Check sheet for the modelled part. Datum: model origin and axes. Units: mm. Face numbers are marked on the shaded views. Round coordinates to 2 decimals unless told otherwise and drop trailing zeros. Loops run counter-clockwise (first coordinate to the right, second up) from the corner with the lowest first, then second, coordinate; pieces in that order, holes last. Notation, with made-up numbers: (-9.5, 28) -> (34.5, 28) arc R16 ccw to (34.5, 36) -> close; hole circle Ø8 at (34.25, -21.75). An arc over 180 degrees is marked (long way). One line per item, written item: value. Start each with the question number.
1. Cross-section at C-C on x = 254.5. Record the cut outline in (y, z), then the cut area to 3 significant figures.
2. Cross-section at B-B on z = 916.5. Record the cut outline in (x, y) (1 decimal).
3. Cross-section at D-D on x = 0. Record the cut outline in (y, z).
4. Material ranges on L1, parallel to Z at x = -1.5, y = 0.05; L2, parallel to Z at x = 63, y = -1.2; L3, parallel to Z at x = 177, y = 0.05, recorded low to high.
5. Go/stop test with flat-tipped pins: pin 1 (1.5 mm diameter, centred on x = 325, y = 0, fed in from +Z); pin 2 (1.6 mm diameter, centred on y = 0.5, z = 890, fed in from +X). Record where each tip stops, or that it passes through.
6. Cross-section at A-A on y = -0.25. Record the cut outline in (x, z) (3 decimals), then the cut area to 3 significant figures.
7. Release check for a two-part mould opening along Y. For the marked faces 1 and 2 record: +Y half, -Y half, draft (parallel to the pull), parting line (faces both ways), or undercut.
from build123d import *

# Parameters (mm, degrees)
BOSS_EXTRUDE1_DEPTH = 1.5875


with BuildPart() as part:
    # Sketch1 → Boss-Extrude1 (new, symmetric)
    with BuildSketch(Plane(origin=(0, 0, 0), x_dir=(1, 0, 0), z_dir=(0, 1, 0))):
        with BuildLine():
            Line((60.325, -1117.6), (525.1196, -749.3))
            Line((525.1196, -749.3), (525.1196, -647.7))
            Line((525.1196, -647.7), (-73.025, -647.7))
            Line((-73.025, -647.7), (-73.025, -1117.6))
            Line((-73.025, -1117.6), (-13.081, -1117.6))
            ThreePointArc((-13.081, -1117.6), (0, -1104.519), (13.081, -1117.6))
            Line((13.081, -1117.6), (60.325, -1117.6))
        make_face()
        Polygon((60.325, -1028.7), (60.325, -704.85), (404.076843973, -704.85), (404.076843973, -756.313435837), align=None, mode=Mode.SUBTRACT)
    extrude(amount=BOSS_EXTRUDE1_DEPTH, both=True)


solid = part.part
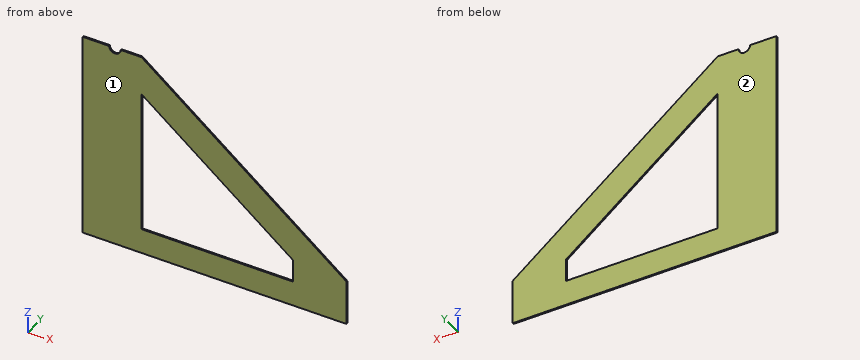
Taken from the geometry:
1. outline: (-1.59, 647.7) -> (1.59, 647.7) -> (1.59, 704.85) -> (-1.59, 704.85) -> close; (-1.59, 874.84) -> (1.59, 874.84) -> (1.59, 963.74) -> (-1.59, 963.74) -> close
1. area: 464 mm2
2. outline: (-73, -1.6) -> (60.3, -1.6) -> (60.3, 1.6) -> (-73, 1.6) -> close; (201.9, -1.6) -> (314.1, -1.6) -> (314.1, 1.6) -> (201.9, 1.6) -> close
3. outline: (-1.59, 647.7) -> (1.59, 647.7) -> (1.59, 1104.52) -> (-1.59, 1104.52) -> close
4. L1: z = 647.7 to 1104.61
4. L2: z = 647.7 to 704.85, 1026.58 to 1115.48
4. L3: z = 647.7 to 704.85, 936.25 to 1025.15
5. pin 1: stops at z = 908.47
5. pin 2: stops at x = 348.57
6. outline: (-73.025, 647.7) -> (525.12, 647.7) -> (525.12, 749.3) -> (60.325, 1117.6) -> (13.081, 1117.6) arc R13.081 cw to (-13.081, 1117.6) -> (-73.025, 1117.6) -> close; hole (60.325, 704.85) -> (404.077, 704.85) -> (404.077, 756.313) -> (60.325, 1028.7) -> close
6. area: 131,000 mm2
7. face 1: -Y half
7. face 2: +Y half
